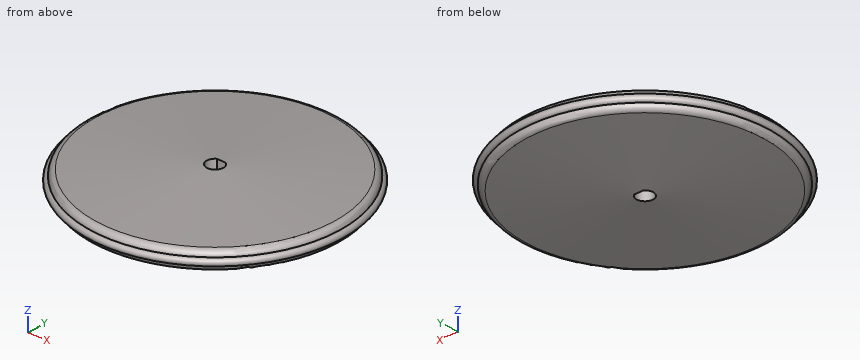
```python
from build123d import *

# Parameters (mm, degrees)
ENL_V_MAT_EXTRU_3_DEPTH      = 64.835726674
ENL_V_MAT_EXTRU_3_DEPTH_BACK = 64.835726674
ESQUISSE4_R                  = 1.3


with BuildPart() as part:
    # Esquisse2 → Révolution1 (revolve)
    with BuildSketch(Plane(origin=(0, 0, 0), x_dir=(0, 0, -1), z_dir=(1, 0, 0)), mode=Mode.PRIVATE) as r_volution1_sk:
        with BuildLine():
            Line((5, 0), (-5, 0))
            Line((-5, 0), (-3.3, 43))
            ThreePointArc((-3.3, 43), (-2.691251544, 44.391251544), (-1.3, 45))
            ThreePointArc((-1.3, 45), (0, 43.7), (1.3, 45))
            ThreePointArc((1.3, 45), (2.691251544, 44.391251544), (3.3, 43))
            Line((3.3, 43), (5, 0))
        make_face()
    revolve(r_volution1_sk.sketch.rotate(Axis((0, 0, 77.254476924), (0, 0, -1)), 90), axis=Axis((0, 0, 77.254476924), (0, 0, -1)))

    # Esquisse3 → Enlèv. mat.-Extru.3 (cut, two sides: drawn at the far end of the back side and taken through both)
    with BuildSketch(Plane.XY.offset(-ENL_V_MAT_EXTRU_3_DEPTH_BACK)):
        with BuildLine():
            Line((-1.658312395, 2.5), (1.658312395, 2.5))
            ThreePointArc((1.658312395, 2.5), (0, -3), (-1.658312395, 2.5))
        make_face()
    extrude(amount=ENL_V_MAT_EXTRU_3_DEPTH + ENL_V_MAT_EXTRU_3_DEPTH_BACK, mode=Mode.SUBTRACT)

    # Esquisse4 → Révolution2 (revolve)
    with BuildSketch(Plane(origin=(0, 0, 0), x_dir=(0, 0, -1), z_dir=(1, 0, 0)), mode=Mode.PRIVATE) as r_volution2_sk:
        with Locations((0, 45)):
            Circle(ESQUISSE4_R)
    revolve(r_volution2_sk.sketch.rotate(Axis((0, 0, 0), (0, 0, -1)), 326.442690238), axis=Axis((0, 0, 0), (0, 0, -1)))


solid = part.part
```
CAD build for the part. Positions are in the model's coordinates, mm. Round coordinates to 2 decimals unless told otherwise and drop trailing zeros. Loops run counter-clockwise (first coordinate to the right, second up) from the corner with the lowest first, then second, coordinate; pieces in that order, holes last. Notation, with made-up numbers: M 10.25,-34 L 54.25,-34 A6 ccw 54.25,-24 Z; hole C 39.25,-27 d10. An arc over 180 degrees is marked long. Use a Markdown table: item, result. Add a question column.
(1) Cut at A-A (x = 0). Give the cut face in (y, z), and give its area (3 significant figures).
(2) Flat gauge pins, fed straight in: pin 1 (8 mm diameter, centred on x = -1, y = 19, fed in from +Z); pin 2 (2 mm diameter, centred on x = -5.5, z = 1, fed in from -Y); pin 3 (1.5 mm diameter, centred on y = -35, z = -3.5, fed in from -X). Where does each tip first touch, or does it go through?
(3) Drill centre lines: line 1 (Y direction, x = 0, z = -2.25); line 2 (Z direction, x = 21, y = -37.5); line 3 (Y direction, x = -40.5, z = -2). Where is each one in solid material? Low to high.
(4) Cut at B-B (y = 0). Give the cut face in (x, z), and give its area (3 significant figures).
(5) Cut at C-C (z = 0). Give the cut face in (x, y).
Geometry says:
| question | item | result |
|---|---|---|
| 1 | outline | M -45,-1.3 A2.08 ccw -43,-3.3 L -3,-4.88 L -3,4.88 L -43,3.3 A2.08 ccw -45,1.3 A1.3 ccw Z; M 2.5,-4.9 L 43,-3.3 A2.08 ccw 45,-1.3 A1.3 ccw 45,1.3 A2.08 ccw 43,3.3 L 2.5,4.9 Z |
| 1 | area | 687 mm² |
| 2 | pin 1 | stops at z = 4.41 |
| 2 | pin 2 | stops at y = -46.02 |
| 2 | pin 3 | stops at x = -27.49 |
| 3 | line 1 | y = -44.73 to -3, 2.5 to 44.73 |
| 3 | line 2 | z = -3.3 to 3.3 |
| 3 | line 3 | y = -19.27 to 19.27 |
| 4 | outline | M -45,-1.3 A2.08 ccw -43,-3.3 L -3,-4.88 L -3,4.88 L -43,3.3 A2.08 ccw -45,1.3 A1.3 ccw Z; M 3,-4.88 L 43,-3.3 A2.08 ccw 45,-1.3 A1.3 ccw 45,1.3 A2.08 ccw 43,3.3 L 3,4.88 Z |
| 4 | area | 683 mm² |
| 5 | outline | C 0,0 d92.6; hole M -1.66,2.5 A3 ccw long 1.66,2.5 Z |
